from build123d import *

# Parameters (mm, degrees)
SKETCH1_R           = 0.635
BOSS_EXTRUDE1_DEPTH = 0.5
SKETCH2_R           = 4.875
BOSS_EXTRUDE2_DEPTH = 4.5


with BuildPart() as part:
    # Sketch1 → Boss-Extrude1 (new body)
    with BuildSketch(Plane(origin=(0, 0, 0), x_dir=(1, 0, 0), z_dir=(0, 1, 0))):
        with BuildLine():
            Line((-5.08, 7.112), (5.08, 7.112))
            ThreePointArc((5.08, 7.112), (6.516840979, 6.516840979), (7.112, 5.08))
            Line((7.112, 5.08), (7.112, -18.288))
            Line((7.112, -18.288), (-7.112, -18.288))
            Line((-7.112, -18.288), (-7.112, 5.08))
            ThreePointArc((-7.112, 5.08), (-6.516840979, 6.516840979), (-5.08, 7.112))
        make_face()
        with Locations(Location((5.08, 5.08, 0), (0, 0, 270))):
            Circle(SKETCH1_R, mode=Mode.SUBTRACT)
        with Locations(Location((-5.08, 5.08, 0), (0, 0, 270))):
            Circle(SKETCH1_R, mode=Mode.SUBTRACT)
    extrude(amount=BOSS_EXTRUDE1_DEPTH)

    # Sketch2 → Boss-Extrude2 (add)
    with BuildSketch(Plane(origin=(0, 0, 0), x_dir=(1, 0, 0), z_dir=(0, 1, 0))):
        with Locations(Location((0, 0, 0), (0, 0, 270))):
            Circle(SKETCH2_R)
    extrude(amount=-BOSS_EXTRUDE2_DEPTH)


solid = part.part
Design review of the part built by this model. Coordinates are the model's own, in mm. A direction names the side the tool comes from. Give positions to 0.01 mm unless a question says otherwise; leave off trailing zeros. Order: outer loops, then holes, each group sorted by start corner. A loop starts at its lowest first (then second) coordinate and runs counter-clockwise, first axis right, second up.
1. Add section B-B, the plane x = 0. State the section outline as (y, z) points (3 decimals), then the cut area to 3 significant figures.
Solution:
outline: (-4.5, -4.875) - (0, -4.875) - (0, -7.112) - (0.5, -7.112) - (0.5, 18.288) - (0, 18.288) - (0, 4.875) - (-4.5, 4.875) - close
area: 56.6 mm2
2. Mouldability with a two-part tool opening along Z and no side actions: class faces 1 (the cylindrical face through (-4.545, 0.246, -4.739)), 2 (the cylindrical face through (-6.533, 0.246, -6.501)), 3 (the flat face through (0, -4.5, 0)) as +Z half, -Z half, draft (parallel to the pull), parting line (faces both ways), or undercut.
Solution:
face 1: undercut
face 2: -Z half
face 3: draft
3. Tool access review of faces 4 (the cylindrical face through (4.834, -2.218, -0.635)), 5 (the flat face through (0, 0.5, 5)): name each direction out of +Z, -Z, +X, -X, +Y, -Y from which nothing blocks a thin tool from reaching the whole face with its end or side.
Solution:
face 4: -Y
face 5: +Z, -Z, +X, -X, +Y
4. Add section C-C, the plane y = -3.55. State the section outline as (x, z) points (3 decimals).
Solution:
outline: circle Ø9.75 at (0, 0)
5. To check wall thickness, follow L1, parallel to X at y = 0.2, z = -5.08 (3 decimals); L2, parallel to Y at x = 6.25, z = 8.25; L3, parallel to Z at x = 2, y = -3.4. State the ranges of each line that lie inside material, in increasing order.
Solution:
L1: x = -7.112 to -5.715, -4.445 to 4.445, 5.715 to 7.112
L2: y = 0 to 0.5
L3: z = -4.45 to 4.45
6. Add section A-A, the plane z = 0. State the section outline as (x, y) points (3 decimals), then the cut area to 3 significant figures.
Solution:
outline: (-7.112, 0) - (-4.875, 0) - (-4.875, -4.5) - (4.875, -4.5) - (4.875, 0) - (7.112, 0) - (7.112, 0.5) - (-7.112, 0.5) - close
area: 51.0 mm2
7. For pin 1 Ø7 at (x, z) = (-1.5, 9.5) entering from -Y; pin 2 Ø1 at (x, y) = (0, -2.5) entering from +Z (3 decimals); pin 3 Ø2 at (x, y) = (4.5, -2.5) entering from +Z; pin 4 Ø1.5 at (x, y) = (-0.5, -0.5) entering from +Z, all flat-tipped, find the tip position at first contact; note any pin that passes through.
Solution:
pin 1: stops at y = 0
pin 2: stops at z = 4.875
pin 3: stops at z = 3.39
pin 4: stops at z = 18.29
8. Add section D-D, the plane z = 5.75. State the section outline as (x, y) points, then the cut area to 3 significant figures.
Solution:
outline: (-7.11, 0) - (7.11, 0) - (7.11, 0.5) - (-7.11, 0.5) - close
area: 7.11 mm2
